Geometry: see drawing. Coordinates: mm, zero at the bounding-box minimum. A direction names the side the tool comes from. Round coordinates to 2 decimals unless told otherwise and drop trailing zeros. Loops run counter-clockwise (first coordinate to the right, second up) from the corner with the lowest first, then second, coordinate; pieces in that order, holes last. Notation, with made-up numbers: (-2, 5.25) - (53, 5.25) arc R26 ccw to (53, 22.25) - close; hole circle Ø8 at (12, 0.5). An arc over 180 degrees is marked (long way). Return JSON: item names as keys, results as strings. Group by question number.
1. Material intervals for probe 1 along Z at (x, y) = (66.4, 2.3); probe 2 along Y at (x, z) = (17.5, 8); probe 3 along Z at (x, y) = (62, 2), sorted ascending.
2. Set-up query: the marked faces 1, 2 and 3. Return all of +Z, -Z, +X, -X, +Y, -Y with unobstructed straight access to the full face (end or side cutting, diameter ignored); none if empty.
3. Draft query along Z for the marked faces 4, 5 and 6. Return one class per face: +Z half, -Z half, draft (parallel to the pull), parting line (faces both ways), or undercut.
4. Section D-D on y = 19.5. Return loops of the section in (x, z).
5. Section C-C on x = 26.5. Return loops of the section in (y, z).
6. Section B-B on z = 6.5. Return loops of the section in (x, y) (1 decimal).
7. Section A-A on x = 62. Return loops of the section in (y, z).
8. First-contact query: pin 1 Ø6 at (x, z) = (69, 13.5) entering from +Y; pin 2 Ø5 at (y, z) = (18.5, 11.5) entering from -X; pin 3 Ø8 at (x, z) = (66.4, 23.495) entering from -Y; pin 4 Ø1 at (x, y) = (58.5, 6) entering from +Z. Flat tips, straight axial feed; report the tip coordinate or a pass-through.
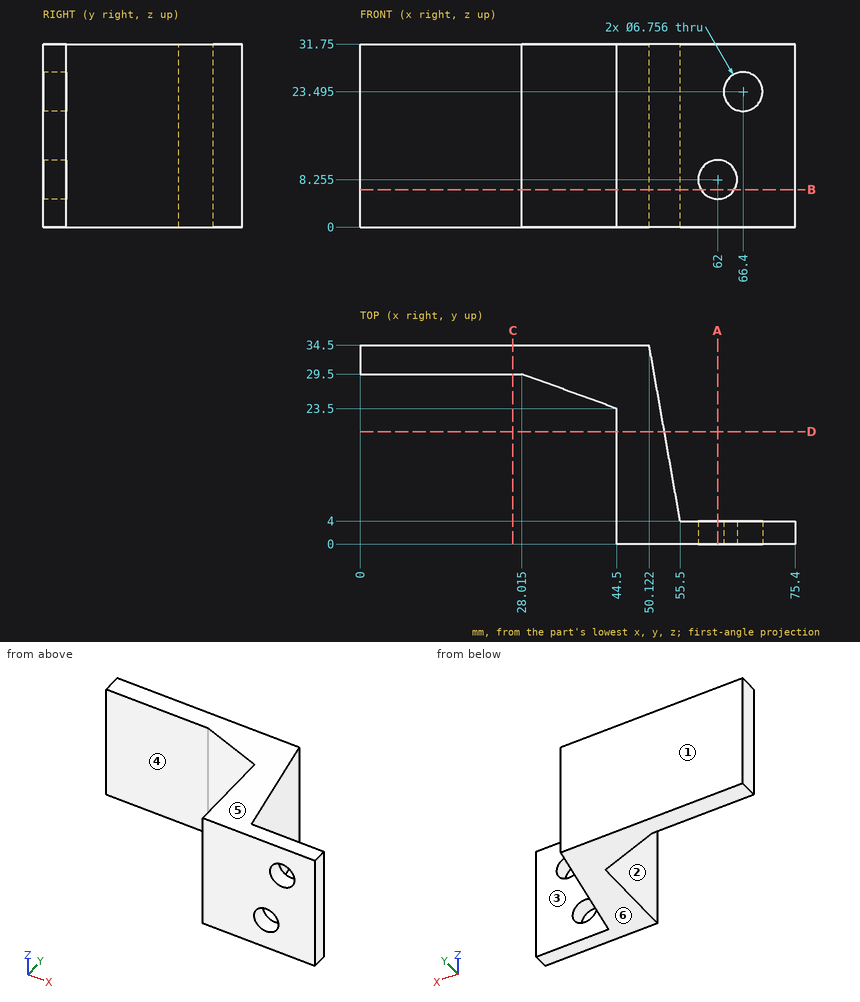
Taken from the geometry:
{
 "1": {"probe 1": "0 to 20.12, 26.87 to 31.75", "probe 2": "29.5 to 34.5", "probe 3": "0 to 4.88, 11.63 to 31.75"},
 "2": {"face 1": "+Z, -Z, +X, -X, +Y", "face 2": "+Z, -Z, -X, -Y", "face 3": "+Z, -Z, +X, +Y"},
 "3": {"face 4": "draft", "face 5": "+Z half", "face 6": "-Z half"},
 "4": {"outline": "(44.5, 0) - (52.77, 0) - (52.77, 31.75) - (44.5, 31.75) - close"},
 "5": {"outline": "(29.5, 0) - (34.5, 0) - (34.5, 31.75) - (29.5, 31.75) - close"},
 "6": {"outline": "(0, 29.5) - (28, 29.5) - (44.5, 23.5) - (44.5, 0) - (59.1, 0) - (59.1, 4) - (55.5, 4) - (50.1, 34.5) - (0, 34.5) - close; (64.9, 0) - (75.4, 0) - (75.4, 4) - (64.9, 4) - close"},
 "7": {"outline": "(0, 0) - (4, 0) - (4, 4.88) - (0, 4.88) - close; (0, 11.63) - (4, 11.63) - (4, 31.75) - (0, 31.75) - close"},
 "8": {"pin 1": "y = 4", "pin 2": "x = 44.5", "pin 3": "y = 0", "pin 4": "through"}
}
